Model file for the job. Use its own axes, mm. Face numbers are marked on the shaded views. A direction names the side the tool comes from. Round coordinates to 2 decimals unless told otherwise and drop trailing zeros. Loops run counter-clockwise (first coordinate to the right, second up) from the corner with the lowest first, then second, coordinate; pieces in that order, holes last. Notation, with made-up numbers: M 80,58 L 117,58 A26 cw 117,83 Z; hole C 35.25,18.25 d7. An arc over 180 degrees is marked long. Use a Markdown table: item, result. Add a question column.
Q1. Mould opens along X. For the marked faces 1, 2 and 3 say: +X half, -X half, draft (parallel to the pull), parting line (faces both ways), or undercut.
Q2. Cut at C-C (x = 60.5). Give the cut face in (y, z), plus the area to 3 significant figures.
Q3. Probe line 1 (X direction, y = 7, z = -25.5); line 2 (Y direction, x = -26.5, z = -15); line 3 (X direction, y = 4.5, z = -3). List the from-to ranges inside material, lowest first. Write a range as from..to.
Q4. Pin check, flat tips, straight feed: pin 1 (20 mm diameter, centred on x = -55.5, z = -21.5, fed in from -Y); pin 2 (6 mm diameter, centred on y = 16, z = 15.5, fed in from +X); pin 3 (1 mm diameter, centred on x = 21, y = -20, fed in from +Z); pin 4 (8 mm diameter, centred on y = -8, z = -22, fed in from +X). Stop position of each tip, or through.
Q5. Cut at A-A (y = 15.5). Give the cut face in (x, z).
Q6. Tool access for the marked faces 4, 5 and 6: list every direction of +Z, -Z, +X, -X, +Y, -Y with a clear straight run to the whole face (end or side of a thin tool).
Q7. Cut at D-D (y = -4). Give the cut face in (x, z), plus the area to 3 significant figures.
Q8. Cut at B-B (z = -26). Give the cut face in (x, y), plus the area to 3 significant figures.
from build123d import *

# Parameters (mm, degrees)
F1_DEPTH      = 7
F1_DEPTH_BACK = 7
F0_R          = 12
F2_DEPTH      = 12
F2_DEPTH_BACK = 12
F3_DEPTH      = 28
F3_DEPTH_BACK = 28
F5_DEPTH      = 57.4
F5_DEPTH_BACK = 40.2
F6_DEPTH      = 102.2
F6_DEPTH_BACK = 32.7


with BuildPart() as f1:
    # F0 (on Front) → F1 (new body, two sides)
    with BuildSketch(Plane.XZ) as f1_sk:
        with BuildLine():
            ThreePointArc((-62.5426396728, -0.7066852599), (-48.400504049, -6.5645496362), (-42.5426396728, -20.7066852599))
            Line((-42.5426396728, -20.7066852599), (32.9624628994, -20.7066852599))
            ThreePointArc((32.9624628994, -20.7066852599), (22.7876905063, -0.5039755893), (27.0942402723, 21.7025347263))
            Line((27.0942402723, 21.7025347263), (-62.5426396728, -0.7066852599))
        make_face()
    extrude(amount=F1_DEPTH)
    extrude(f1_sk.sketch, amount=-F1_DEPTH_BACK)

    # F0 (on Front) → F2 (join, two sides)
    with BuildSketch(Plane.XZ) as f2_sk:
        with BuildLine():
            ThreePointArc((-62.5426396728, -0.7066852599), (-76.6847752965, -34.8488208837), (-42.5426396728, -20.7066852599))
            ThreePointArc((-42.5426396728, -20.7066852599), (-48.400504049, -6.5645496362), (-62.5426396728, -0.7066852599))
        make_face()
        with Locations((-62.5426396728, -20.7066852599)):
            Circle(F0_R, mode=Mode.SUBTRACT)
    extrude(amount=F2_DEPTH)
    extrude(f2_sk.sketch, amount=-F2_DEPTH_BACK)

    # F0 (on Front) → F3 (join, two sides)
    with BuildSketch(Plane.XZ) as f3_sk:
        with BuildLine():
            ThreePointArc((27.0942402723, 21.7025347263), (22.7876905063, -0.5039755893), (32.9624628994, -20.7066852599))
            ThreePointArc((32.9624628994, -20.7066852599), (71.0160953351, -27.9737072017), (92.4573603272, 4.2933147401))
            ThreePointArc((92.4573603272, 4.2933147401), (66.4654344299, 38.114234316), (27.0942402723, 21.7025347263))
        make_face()
        with BuildLine():
            ThreePointArc((57.4573603272, 29.2933147401), (75.1350298569, 21.9709842697), (82.4573603272, 4.2933147401))
            ThreePointArc((82.4573603272, 4.2933147401), (75.1350298569, -13.3843547896), (57.4573603272, -20.7066852599))
            ThreePointArc((57.4573603272, -20.7066852599), (39.7796907976, -13.3843547896), (32.4573603272, 4.2933147401))
            ThreePointArc((32.4573603272, 4.2933147401), (39.7796907976, 21.9709842697), (57.4573603272, 29.2933147401))
        make_face(mode=Mode.SUBTRACT)
    extrude(amount=F3_DEPTH)
    extrude(f3_sk.sketch, amount=-F3_DEPTH_BACK)

    # F4 (on face) → F5 (cut, two sides)
    with BuildSketch(Plane.XZ) as f5_sk:
        with BuildLine():
            ThreePointArc((32.9624628994, -0.7066852599), (32.5839565021, 1.7805906899), (32.4573603272, 4.2933147401))
            Line((32.4573603272, 4.2933147401), (28.4573603272, 4.2933147401))
            Line((28.4573603272, 4.2933147401), (28.4573603272, -0.7066852599))
            Line((28.4573603272, -0.7066852599), (32.9624628994, -0.7066852599))
        make_face()
    extrude(amount=-F5_DEPTH, mode=Mode.SUBTRACT)
    extrude(f5_sk.sketch, amount=F5_DEPTH_BACK, mode=Mode.SUBTRACT)

    # F4 (on face) → F6 (cut, two sides)
    with BuildSketch(Plane.XZ) as f6_sk:
        with BuildLine():
            Line((28.4573603272, 4.2933147401), (32.4573603272, 4.2933147401))
            ThreePointArc((32.4573603272, 4.2933147401), (32.5839565021, 6.8060387902), (32.9624628994, 9.2933147401))
            Line((32.9624628994, 9.2933147401), (32.4573603272, 9.2933147401))
            Line((32.4573603272, 9.2933147401), (28.4573603272, 9.2933147401))
            Line((28.4573603272, 9.2933147401), (28.4573603272, 4.2933147401))
        make_face()
    extrude(amount=-F6_DEPTH, mode=Mode.SUBTRACT)
    extrude(f6_sk.sketch, amount=F6_DEPTH_BACK, mode=Mode.SUBTRACT)


solid = f1.part
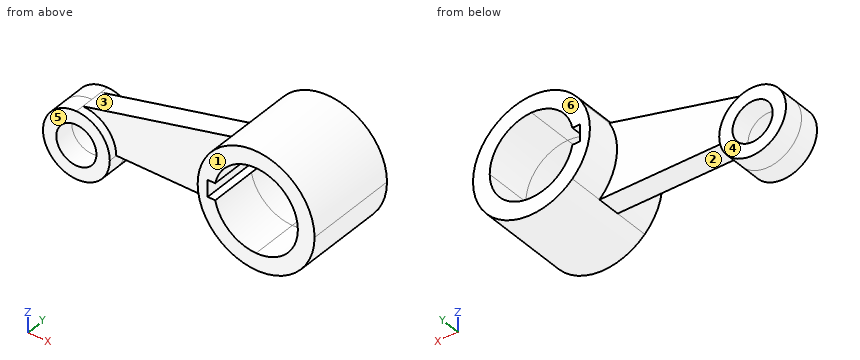
Checked values:
| question | item | result |
|---|---|---|
| 1 | face 1 | draft |
| 1 | face 2 | undercut |
| 1 | face 3 | -X half |
| 2 | outline | M -28,-30.57 L 28,-30.57 L 28,-20.52 L -28,-20.52 Z; M -28,29.11 L 28,29.11 L 28,39.16 L -28,39.16 Z |
| 2 | area | 1,130 mm^2 |
| 3 | line 1 | x = -81.96..-73.54, -51.54..-43.13, 39.09..75.82 |
| 3 | line 2 | y = -7..7 |
| 3 | line 3 | x = -71.84..33.54, 81.37..91.69 |
| 4 | pin 1 | stops at y = -12 |
| 4 | pin 2 | stops at x = 91.48 |
| 4 | pin 3 | passes through |
| 4 | pin 4 | stops at x = 84.44 |
| 5 | outline | C 57.46,4.29 d70; hole M 28.46,-0.71 L 32.96,-0.71 A25 ccw long 32.96,9.29 L 28.46,9.29 Z |
| 6 | face 4 | +Z, -Z, -X, +Y |
| 6 | face 5 | +Z, -Z, -X, -Y |
| 6 | face 6 | +Z, -Z, +X, -X, +Y |
| 7 | outline | M -62.54,-0.71 A20 ccw long -42.54,-20.71 L 32.96,-20.71 A35 ccw long 27.09,21.7 Z; hole C -62.54,-20.71 d24; hole M 28.46,-0.71 L 32.96,-0.71 A25 ccw long 32.96,9.29 L 28.46,9.29 Z |
| 7 | area | 5,040 mm^2 |
| 8 | outline | M -81.83,-12 L -73.31,-12 L -73.31,12 L -81.83,12 Z; M -51.77,-12 L -43.26,-12 L -43.26,12 L -51.77,12 Z; M 39.93,-28 L 74.99,-28 L 74.99,28 L 39.93,28 Z |
| 8 | area | 2,370 mm^2 |
